Autodesk Inventor part; units mm, degrees
ref_plane "YZ Plane" through (0, 0, 0) normal (1, 0, 0) x (0, 1, 0)
ref_plane "XZ Plane" through (0, 0, 0) normal (0, 1, 0) x (-1, 0, 0)
ref_plane "XY Plane" through (0, 0, 0) normal (0, 0, 1) x (1, 0, 0)
sketch "스케치1" plane through (0, 0, 0) normal (0, 0, 1) x (1, 0, 0)
  circle A0 centre (0, 0) radius 2.5
  line L0 (0, 0) -> (0, 40)
  line L1 (4, 6) -> (4, -4)
  line L2 (4, -4) -> (-4, -4)
  line L3 (-4, -4) -> (-4, 6)
  line L4 (-6, 32) -> (6, 32)
  line L5 (6, 32) -> (6, 11)
  line L6 (-6, 11) -> (-6, 32)
  line L7 (-6, 11) -> (-4, 6)
  line L8 (6, 11) -> (4, 6)
  dimension "d0" = 5
  dimension "d1" = 40
  dimension "d2" = 8
  dimension "d3" = 4
  dimension "d4" = 4
  dimension "d5" = 36
  dimension "d8" = 12
  dimension "d9" = 6
  dimension "d10" = 10
  dimension "d11" = 5
  dimension "d12" = 5
  dimension "d13" = 10
extrude "돌출1" add sketch "스케치1" along normal blind 5
extrude "돌출2" add sketch "스케치1" along normal blind 15 contours A0
sketch "스케치2" plane through (0, 0, 0) normal (0, 0, -1) x (-1, 0, 0)
  circle A0 centre (0, 26) radius 2.5
  line L0 (-6, 11) -> (-6, 32)
  line L1 (4, -4) -> (-4, -4)
  point P0 (0, 0)
  dimension "d18" = 5
  dimension "d19" = 6
  dimension "d20" = 30
extrude "돌출3" add sketch "스케치2" along normal blind 11
sketch "스케치3" plane through (0, 26, -11) normal (0, 0, -1) x (-1, 0, 0)
  circle A0 centre (0, 0) radius 7
  point P0 (0, -26)
  dimension "d23" = 14
extrude "돌출4" add sketch "스케치3" along normal blind 4
fillet "모깎기1" radius 2 2 edges at (-4, -4, 2.5) (4, -4, 2.5)
fillet "모깎기2" radius 6 2 edges at (6, 32, 2.5) (-6, 32, 2.5)
properties part number "2번부품"
Can you work these out from the model? Positions are in its coordinate system, mm. A direction names the side the tool comes from. Round coordinates to 2 decimals unless told otherwise and drop trailing zeros. Loops run counter-clockwise (first coordinate to the right, second up) from the corner with the lowest first, then second, coordinate; pieces in that order, holes last. Notation, with made-up numbers: M -21,29.5 L 34,29.5 A16 ccw 34,45.5 Z; hole C -38.75,-1.5 d4. An arc over 180 degrees is marked long. Answer in a Markdown table with one row per item.
1. If we section it at B-B, the plane x = -5.5: Please give me the cut outline in (y, z), plus the area to 3 significant figures.
Established:
| item | result |
|---|---|
| outline | M 9.75,0 L 28.4,0 L 28.4,5 L 9.75,5 Z; M 21.67,-15 L 30.33,-15 L 30.33,-11 L 21.67,-11 Z |
| area | 128 mm² |
2. On a 3-axis mill with a long thin cutter (end or side, diameter ignored), from which of +Z, -Z, +X, -X, +Y, -Y can I reach the whole of each face in a straight line? I mean faces 1 (the face through (-4.196, 30.289, 2.535)), 2 (the face through (1.517, 32.834, -12.972)), 3 (the face through (0.33, 23.52, -5.42)). Say none if no direction works.
Established:
| item | result |
|---|---|
| face 1 | +Z, -X, +Y |
| face 2 | -Z |
| face 3 | none |
3. If we section it at D-D, the plane x = 1.25: Please give me the cut outline in (y, z), plus the area to 3 significant figures.
Established:
| item | result |
|---|---|
| outline | M -4,0 L 23.83,0 L 23.83,-11 L 19.11,-11 L 19.11,-15 L 32.89,-15 L 32.89,-11 L 28.17,-11 L 28.17,0 L 31.87,0 L 31.87,5 L 2.17,5 L 2.17,15 L -2.17,15 L -2.17,5 L -4,5 Z |
| area | 325 mm² |
4. Thinking about a two-plate mould opening in Z: for faces 4 (the face through (0, 0, 15)), 5 (the face through (5, 8.5, 2.5)), 6 (the face through (-3, 26, -11)), which applies, pulls with the +Z half, pulls with the -Z half, needs draft (parallel to the pull), parting line crosses it, or undercut?
Established:
| item | result |
|---|---|
| face 4 | pulls with the +Z half |
| face 5 | needs draft |
| face 6 | undercut |
5. Please list where these lines run through material, in increasing order: line 1 (Z direction, x = -3, y = 26); line 2 (Z direction, x = -0.25, y = 27.5); line 3 (X direction, y = 5, z = 2.25). Write a range as from..to.
Established:
| item | result |
|---|---|
| line 1 | -15..-11, 0..5 |
| line 2 | -15..5 |
| line 3 | -4..4 |
6. I'm going to push flat-ended pins straight in: pin 1 Ø5 at (x, y) = (-5.5, 20) entering from +Z; pin 2 Ø1.5 at (x, y) = (-3.5, 2.5) entering from -Z; pin 3 Ø1.5 at (y, z) = (16.5, 1.5) entering from +X. Where does each tip first touch, or does it pass through?
Established:
| item | result |
|---|---|
| pin 1 | z = 5 |
| pin 2 | z = 0 |
| pin 3 | x = 6 |
7. If we section it at C-C, the plane y = 0: Please give me the cut outline in (x, z), plus the area to 3 significant figures.
Established:
| item | result |
|---|---|
| outline | M -4,0 L 4,0 L 4,5 L 2.5,5 L 2.5,15 L -2.5,15 L -2.5,5 L -4,5 Z |
| area | 90.0 mm² |
